Source: CAD feature listing. Evaluate the final solid. Frame: model axes, mm. A direction names the side the tool comes from. Round coordinates to 2 decimals unless told otherwise and drop trailing zeros. Order: outer loops, then holes, each group sorted by start corner. A loop starts at its lowest first (then second) coordinate and runs counter-clockwise, first axis right, second up.
Autodesk Inventor part; units mm, degrees
ref_plane "YZ Plane" through (0, 0, 0) normal (1, 0, 0) x (0, 1, 0)
ref_plane "XZ Plane" through (0, 0, 0) normal (0, 1, 0) x (-1, 0, 0)
ref_plane "XY Plane" through (0, 0, 0) normal (0, 0, 1) x (1, 0, 0)
sketch "Boceto1" plane through (0, 0, 0) normal (0, 1, 0) x (-1, 0, 0)
  line L0 (105, 200) -> (-105, 200)
  line L1 (-105, 200) -> (-105, -200)
  line L2 (-105, -200) -> (105, -200)
  line L3 (105, -200) -> (105, 200)
  line L4 (105, 200) -> (-105, -200) construction
  line L5 (-105, 200) -> (105, -200) construction
  point P0 (0, 0)
  dimension "d0" = 210
  dimension "d1" = 400
extrude "Extrusión1" add sketch "Boceto1" along normal blind 120
sketch "Boceto2" plane through (0, 120, 0) normal (0, 1, 0) x (1, 0, 0)
  line L0 (-85, -180) -> (85, -180)
  line L1 (85, -180) -> (85, 180)
  line L2 (85, 180) -> (-85, 180)
  line L3 (-85, 180) -> (-85, -180)
  line L4 (-85, -180) -> (85, 180) construction
  line L5 (85, -180) -> (-85, 180) construction
  point P0 (0, 0)
  dimension "d4" = 170
  dimension "d5" = 360
extrude "Extrusión2" cut sketch "Boceto2" against normal blind 100
sketch "Boceto3" plane through (0, 0, 0) normal (0, -1, 0) x (1, 0, 0)
  line L0 (105, 143) -> (75, 143)
  line L1 (75, 143) -> (75, 123)
  line L2 (75, 123) -> (105, 123)
  line L3 (105, 123) -> (105, 143)
  line L4 (105, 143) -> (75, 123) construction
  line L5 (75, 143) -> (105, 123) construction
  line L6 (105, -140) -> (75, -140)
  line L7 (75, -140) -> (75, -160)
  line L8 (75, -160) -> (105, -160)
  line L9 (105, -160) -> (105, -140)
  line L10 (105, -140) -> (75, -160) construction
  line L11 (75, -140) -> (105, -160) construction
  line L12 (105, -200) -> (-105, -200)
  line L13 (-105, 143) -> (-75, 143)
  line L14 (-75, 143) -> (-75, 123)
  line L15 (-75, 123) -> (-105, 123)
  line L16 (-105, 123) -> (-105, 143)
  line L17 (-105, 143) -> (-75, 123) construction
  line L18 (-75, 143) -> (-105, 123) construction
  line L19 (-105, -140) -> (-75, -140)
  line L20 (-75, -140) -> (-75, -160)
  line L21 (-75, -160) -> (-105, -160)
  line L22 (-105, -160) -> (-105, -140)
  line L23 (-105, -140) -> (-75, -160) construction
  line L24 (-75, -140) -> (-105, -160) construction
  line L25 (-105, 200) -> (105, 200)
  point P0 (0, 0)
  point P1 (90, 133)
  point P2 (105, 133)
  point P3 (90, -150)
  point P4 (105, -150)
  point P5 (-90, 35)
  point P6 (-105, 35)
  point P7 (-90, -150)
  point P8 (-105, -150)
  point P9 (-90, 143)
  dimension "d9" = 20
  dimension "d12" = 20
  dimension "d34" = 57
  dimension "d35" = 57
  dimension "d36" = 20
  dimension "d37" = 40
  dimension "d38" = 40
extrude "Extrusión3" add sketch "Boceto3" along normal blind 90
sketch "Boceto6" plane through (-75, 0, 143) normal (1, 0, 0) x (0, 0, -1)
  line L0 (0, 0) -> (0, -90)
  line L1 (20, 0) -> (20, -90)
  line L2 (0, -90) -> (20, -90)
  line L3 (20, -90) -> (20, -80)
  line L4 (20, -80) -> (0, -80)
  line L5 (0, -80) -> (0, -90)
  point P0 (143, 0)
  dimension "d16" = 10
extrude "Extrusión4" add sketch "Boceto6" along normal blind 150
sketch "Boceto7" plane through (-75, 0, -140) normal (1, 0, 0) x (0, 0, -1)
  line L0 (0, 0) -> (0, -90)
  line L1 (20, 0) -> (20, -90)
  line L2 (0, -90) -> (20, -90)
  line L3 (20, -90) -> (20, -80)
  line L4 (20, -80) -> (0, -80)
  line L5 (0, -80) -> (0, -90)
  point P0 (-140, 0)
  dimension "d19" = 10
extrude "Extrusión5" add sketch "Boceto7" along normal blind 150
sketch "Boceto8" plane through (0, -90, 0) normal (0, -1, 0) x (1, 0, 0)
  circle A0 centre (-65, 133) radius 5
  circle A1 centre (65, 133) radius 5
  line L0 (-105, 143) -> (-105, 123)
  line L1 (105, 123) -> (105, 143)
  line L2 (60, 123) -> (60, 143)
  line L3 (105, 143) -> (-105, 143)
  point P0 (0, 0)
  dimension "d22" = 10
  dimension "d23" = 10
  dimension "d24" = 40
  dimension "d25" = 40
  dimension "d39" = 10
  dimension "d40" = 10
sketch "Boceto9" plane through (0, -90, 0) normal (0, -1, 0) x (1, 0, 0)
  circle A0 centre (-65, -150) radius 5
  circle A1 centre (65, -150) radius 5
  line L0 (-105, -140) -> (-105, -160)
  line L1 (105, -160) -> (105, -140)
  point P0 (0, 0)
  dimension "d26" = 10
  dimension "d27" = 10
  dimension "d28" = 40
  dimension "d29" = 40
extrude "Extrusión6" cut sketch "Boceto8" against normal blind 20
extrude "Extrusión7" cut sketch "Boceto9" against normal blind 20
properties part number "container"
1. Line query: line 1 along Z through (x, y) = (65, -83.5); line 2 along Z through (x, y) = (-17, 102); line 3 along X through (y, z) = (24.5, 119). Output: solid intervals per line, ascending.
2. Section A-A on y = -6.5. Return loops of the section in (x, z), plus the area to 3 significant figures.
3. First-contact query: pin 1 (10 mm diameter, centred on x = 5.5, z = 137, fed in from +Y); pin 2 (12 mm diameter, centred on x = 72.5, y = -16, fed in from -Z). Flat tips, straight axial feed; report the tip coordinate or a pass-through.
4. Access query for faces 1 (the face through (-85, 71, -3)), 2 (the face through (7, -81, -140)), 3 (the face through (75, -39, -150)). Directions: +Z, -Z, +X, -X, +Y, -Y. A direction counts if a zero-diameter tool reaches every point of the face in a straight line with its end or side. Return the directions, or none.
5. Section D-D on z = 86. Return loops of the section in (x, y).
6. Section C-C on z = -150. Return loops of the section in (x, y), plus the area to 3 significant figures.
7. Section B-B on x = -14. Return loops of the section in (y, z).
8. Pull-direction query (Y, two-part tool) for faces 4 (the face through (-1, 20, -3)), 5 (the face through (-1, -80, -150)), 6 (the face through (-1, 71, 180)), 7 (the face through (-1, -90, -150)); classes: released by +Y, released by -Y, zero draft, split by the parting line, or undercut.
Result:
1. line 1: z = -160 to -155, -145 to -140, 123 to 128, 138 to 143
1. line 2: z = -200 to -180, 180 to 200
1. line 3: x = -105 to -85, 85 to 105
2. outline: (-105, -160) - (-75, -160) - (-75, -140) - (-105, -140) - close; (-105, 123) - (-75, 123) - (-75, 143) - (-105, 143) - close; (75, -160) - (105, -160) - (105, -140) - (75, -140) - close; (75, 123) - (105, 123) - (105, 143) - (75, 143) - close
2. area: 2,400 mm2
3. pin 1: stops at y = 20
3. pin 2: stops at z = -160
4. face 1: +Y
4. face 2: +X, -X, -Y
4. face 3: +Z, -Z
5. outline: (-105, 0) - (105, 0) - (105, 120) - (85, 120) - (85, 20) - (-85, 20) - (-85, 120) - (-105, 120) - close
6. outline: (-105, -90) - (-70, -90) - (-70, -80) - (-75, -80) - (-75, 0) - (75, 0) - (75, -80) - (70, -80) - (70, -90) - (105, -90) - (105, 120) - (85, 120) - (85, 20) - (-85, 20) - (-85, 120) - (-105, 120) - close; (-60, -90) - (60, -90) - (60, -80) - (-60, -80) - close
6. area: 14,900 mm2
7. outline: (-90, -160) - (-80, -160) - (-80, -140) - (-90, -140) - close; (-90, 123) - (-80, 123) - (-80, 143) - (-90, 143) - close; (0, -200) - (120, -200) - (120, -180) - (20, -180) - (20, 180) - (120, 180) - (120, 200) - (0, 200) - close
8. face 4: released by +Y
8. face 5: undercut
8. face 6: zero draft
8. face 7: released by -Y
